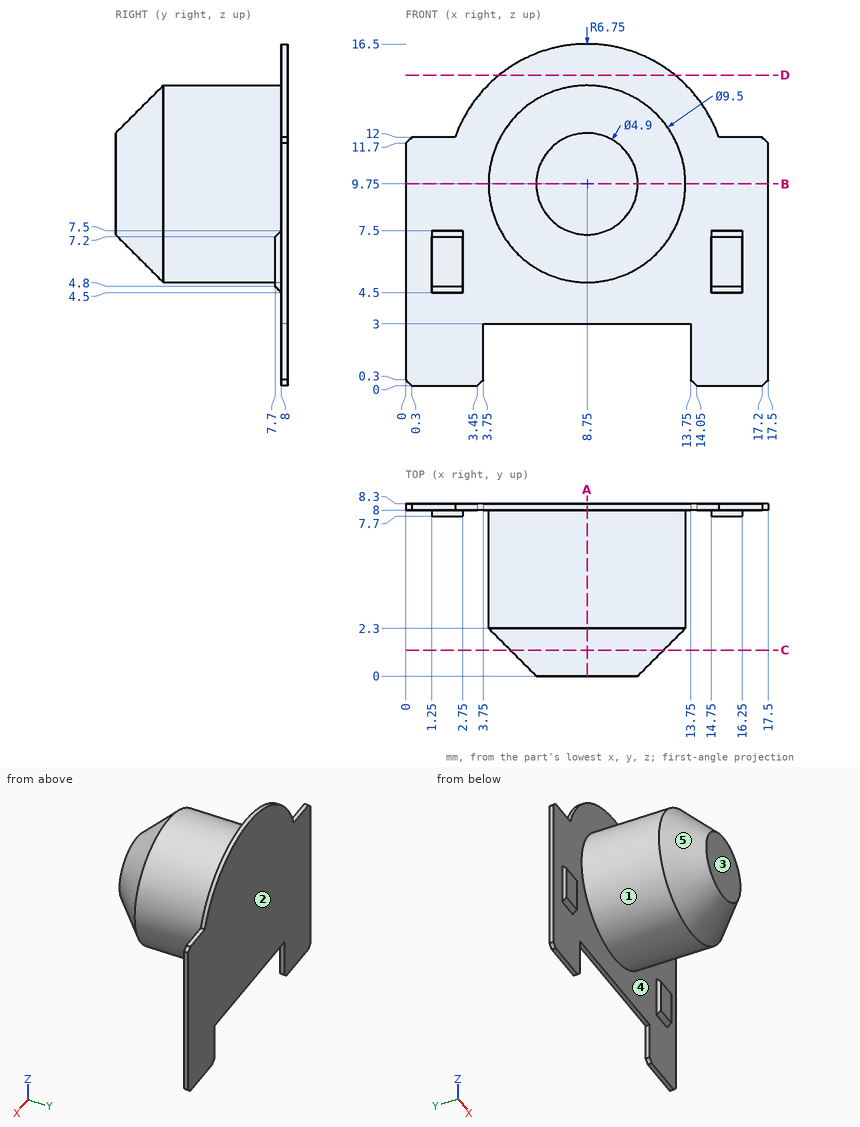
Job drawing, mm, ordinate dimensions from the low corner. One solid piece. A direction names the side the tool comes from. Round coordinates to 2 decimals unless told otherwise and drop trailing zeros. Order: outer loops, then holes, each group sorted by start corner. A loop starts at its lowest first (then second) coordinate and runs counter-clockwise, first axis right, second up. Notation, with made-up numbers: (60, 47.25) -> (76, 47.25) arc R20 cw to (76, 81.25) -> close; hole circle Ø3 at (-17.5, -27.5). An arc over 180 degrees is marked (long way). Answer in a Markdown table with one row per item.
1) Wall check: L1, parallel to Y at x = 13.5, z = 13.5; L2, parallel to Y at x = 5.75, z = 10.5; L3, parallel to X at y = 6.75, z = 9.5. Give the ranges that are in metal, low to high.
Values:
| item | result |
|---|---|
| L1 | 8 to 8.3 |
| L2 | 0.64 to 8.3 |
| L3 | 4.01 to 13.49 |
2) Band-saw the part on D-D on z = 15. Give the cut face in (x, y), and give its area (3 significant figures).
Values:
| item | result |
|---|---|
| outline | (4.51, 8) -> (12.99, 8) -> (12.99, 8.3) -> (4.51, 8.3) -> close |
| area | 2.55 mm2 |
3) Band-saw the part on B-B on z = 9.75. Give the cut face in (x, y), and give its area (3 significant figures).
Values:
| item | result |
|---|---|
| outline | (0, 8) -> (4, 8) -> (4, 2.3) -> (6.3, 0) -> (11.2, 0) -> (13.5, 2.3) -> (13.5, 8) -> (17.5, 8) -> (17.5, 8.3) -> (0, 8.3) -> close |
| area | 76.0 mm2 |
4) Which spindle directions (+Z, -Z, +X, -X, +Y, -Y) get a long thin tool onto all of the face, cutting with end or side? Do the marked faces 1 and 2. Say none if no direction does.
Values:
| item | result |
|---|---|
| face 1 | -Y |
| face 2 | +Z, -Z, +X, -X, +Y |
5) Band-saw the part on A-A on x = 8.75. Give the cut face in (y, z), and give its area (3 significant figures).
Values:
| item | result |
|---|---|
| outline | (0, 7.3) -> (2.3, 5) -> (8, 5) -> (8, 3) -> (8.3, 3) -> (8.3, 16.5) -> (8, 16.5) -> (8, 14.5) -> (2.3, 14.5) -> (0, 12.2) -> close |
| area | 74.8 mm2 |
6) Mould opens along X. For the marked faces 3, 4 and 5 say: released by +X, released by -X, zero draft, split by the parting line, or undercut.
Values:
| item | result |
|---|---|
| face 3 | zero draft |
| face 4 | undercut |
| face 5 | split by the parting line |
7) Pin check, flat tips, straight feed: P1, Ø3, axis at x = 3, y = 3.5, coming from the +Z side; P2, Ø5, axis at x = 10.5, z = 5.5, coming from the -Y side; P3, Ø0.8, axis at x = 15.5, z = 6.5, coming from the -Y side; P4, Ø4, axis at x = 7.5, y = 2, coming from the +Z side. Stop position of each tip, or through.
Values:
| item | result |
|---|---|
| P1 | z = 11.87 |
| P2 | y = 0 |
| P3 | y = 7.7 |
| P4 | z = 14.5 |
8) Band-saw the part on C-C on y = 1.25. Give the cut face in (x, z).
Values:
| item | result |
|---|---|
| outline | circle Ø7.4 at (8.75, 9.75) |
